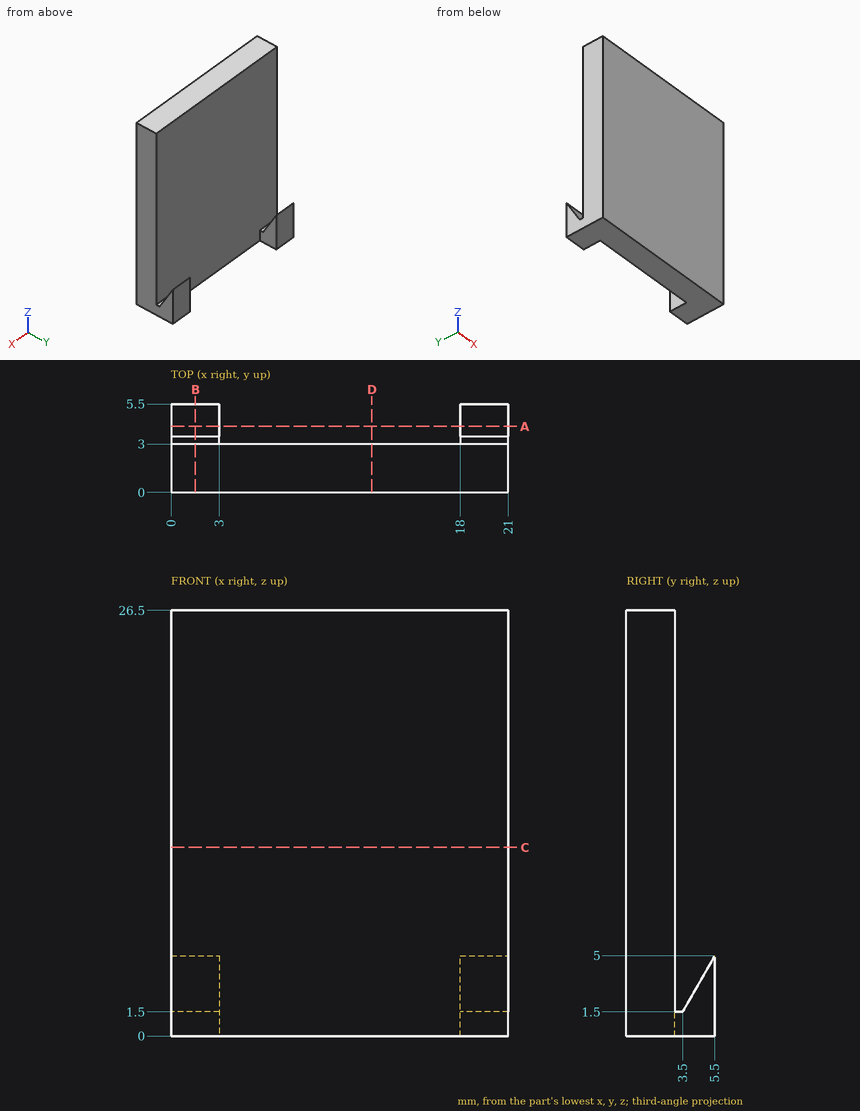
Answer from the drawing. Dimensions are ordinates in mm from the lowest x, y and z of the part. Coordinates: 2 decimals unless noted, no trailing zeros. Loops run counter-clockwise (first coordinate to the right, second up) from the corner with the lowest first, then second, coordinate; pieces in that order, holes last. Notation, with made-up numbers: (-5, 12) -> (49, 12) arc R7 cw to (49, 24) -> close; hole circle Ø9 at (-34, -7). An arc over 180 degrees is marked (long way). Answer in a Markdown table with one row per item.
Item 1: A cutting plane is placed at C-C on z = 11.75. Determine the outline of the cut face in (x, y).
Returned:
| item | result |
|---|---|
| outline | (0, 0) -> (21, 0) -> (21, 3) -> (0, 3) -> close |
Item 2: Straight lines are drawn through the part: line 1 along Y through (x, z) = (13.5, 9.25); line 2 along Z through (x, y) = (1.75, 3.1); line 3 along Z through (x, y) = (1.5, 4.65). For each, find the intervals that lie inside material, in ascending order. Write a range as [from, to].
Returned:
| item | result |
|---|---|
| line 1 | y = [0, 3] |
| line 2 | z = [0, 1.5] |
| line 3 | z = [0, 3.51] |
Item 3: A cutting plane is placed at D-D on x = 12.5. Determine the outline of the cut face in (y, z).
Returned:
| item | result |
|---|---|
| outline | (0, 0) -> (3, 0) -> (3, 26.5) -> (0, 26.5) -> close |
Item 4: A cutting plane is placed at A-A on y = 4.1. Determine the outline of the cut face in (x, z).
Returned:
| item | result |
|---|---|
| outline | (0, 0) -> (3, 0) -> (3, 2.55) -> (0, 2.55) -> close; (18, 0) -> (21, 0) -> (21, 2.55) -> (18, 2.55) -> close |
Item 5: A cutting plane is placed at B-B on x = 1.5. Determine the outline of the cut face in (y, z), plus the area to 4 significant figures.
Returned:
| item | result |
|---|---|
| outline | (0, 0) -> (5.5, 0) -> (5.5, 5) -> (3.5, 1.5) -> (3, 1.5) -> (3, 26.5) -> (0, 26.5) -> close |
| area | 86.75 mm^2 |
